Source: CAD feature listing. Evaluate the final solid. Frame: model axes, mm. Face numbers are marked on the shaded views. A direction names the side the tool comes from. Coordinates: 2 decimals unless noted, no trailing zeros. Loops run counter-clockwise (first coordinate to the right, second up) from the corner with the lowest first, then second, coordinate; pieces in that order, holes last. Notation, with made-up numbers: (71, 50) -> (104, 50) arc R13 cw to (104, 62) -> close; hole circle Ø6 at (-22, 62.5). An arc over 180 degrees is marked (long way). One line per question, with ' | ' between items. Start each with the question number.
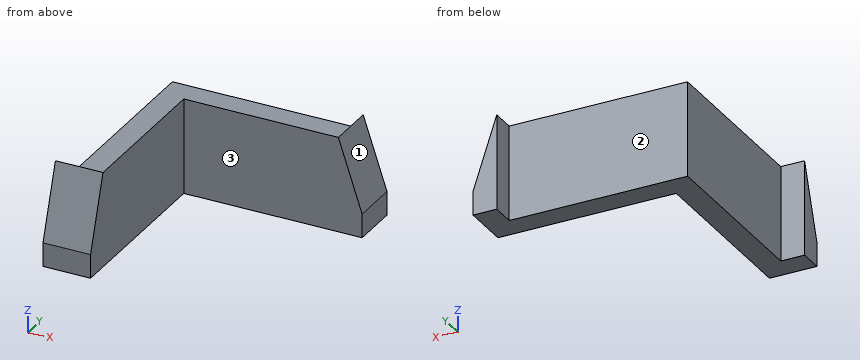
```python
from build123d import *

# Parameters (mm, degrees)
F1_DEPTH = 25.4
F2_SIZE2 = 19.05
F2_SIZE  = 6.35
F5_DEPTH = 6.35
F6_DEPTH = 6.35


with BuildPart() as f1:
    # F0 (on Top) → F1 (new body)
    with BuildSketch(Plane.XY):
        Polygon((-31.75, -22.225), (-25.4, -22.225), (-25.4, 25.4), (22.225, 25.4), (22.225, 31.75), (-31.75, 31.75), align=None)
    extrude(amount=F1_DEPTH)

    # F2
    f2_edges = [f1.edges().sort_by_distance(p)[0] for p in [
        (-28.575, -22.225, 25.4),
        (22.225, 28.575, 25.4),
    ]]
    f2_side = f1.faces().sort_by_distance((-28.575, -21.461678, 25.4))[0]
    chamfer(f2_edges, length=F2_SIZE, length2=F2_SIZE2, reference=f2_side)

    # F4 (on face) → F5 (join)
    with BuildSketch(Plane(origin=(0, 31.75, 0), x_dir=(-1, 0, 0), z_dir=(0, 1, 0))):
        Polygon((-15.875, 0), (-15.875, 25.4), (-22.225, 6.35), (-22.225, 0), align=None)
    extrude(amount=F5_DEPTH)

    # F3 (on face) → F6 (join)
    with BuildSketch(Plane(origin=(-31.75, 0, 0), x_dir=(0, -1, 0), z_dir=(-1, 0, 0))):
        Polygon((22.225, 6.35), (15.875, 25.4), (15.875, 0), (22.225, 0), align=None)
    extrude(amount=F6_DEPTH)


solid = f1.part
```
(1) Cut plane D-D, the plane z = 8.5. Return the cut outline in (x, y) (3 decimals).
(2) Cut plane C-C, the plane y = 14.5. Return the cut outline in (x, z), and give its area (3 significant figures).
(3) Cut plane A-A, the plane z = 4.5. Return the cut outline in (x, y) (3 decimals).
(4) Contact query for flat-ended pins moving along their axis: pin 1 Ø4 at (x, z) = (0, 11) entering from -Y; pin 2 Ø12.5 at (y, z) = (16.5, 8.5) entering from -X; pin 3 Ø3 at (y, z) = (24.5, 4) entering from +X (3 decimals); pin 4 Ø5 at (y, z) = (-11, 15.5) entering from +X. Output: stop coordinate, or through.
(5) Ray query, L1, parallel to X at y = -5, z = 22; L2, parallel to Y at x = 8, z = 19.5; L3, parallel to Y at x = -33.5, z = 5.75 (3 decimals). Return the intervals inside material, ascending.
(6) Cut plane B-B, the plane x = -29. Return the cut outline in (y, z) (3 decimals).
(7) Access query for the marked faces 1, 2 and 3. Directions: +Z, -Z, +X, -X, +Y, -Y. A direction counts if a zero-diameter tool reaches every point of the face in a straight line with its end or side. Return the directions, or none.
Here are the results:
1) outline: (-38.1, -21.508) -> (-25.4, -21.508) -> (-25.4, 25.4) -> (21.508, 25.4) -> (21.508, 38.1) -> (15.875, 38.1) -> (15.875, 31.75) -> (-31.75, 31.75) -> (-31.75, -15.875) -> (-38.1, -15.875) -> close
2) outline: (-31.75, 0) -> (-25.4, 0) -> (-25.4, 25.4) -> (-31.75, 25.4) -> close | area: 161 mm2
3) outline: (-38.1, -22.225) -> (-25.4, -22.225) -> (-25.4, 25.4) -> (22.225, 25.4) -> (22.225, 38.1) -> (15.875, 38.1) -> (15.875, 31.75) -> (-31.75, 31.75) -> (-31.75, -15.875) -> (-38.1, -15.875) -> close
4) pin 1: stops at y = 25.4 | pin 2: stops at x = -31.75 | pin 3: stops at x = 22.225 | pin 4: stops at x = -25.4
5) L1: x = -31.75 to -25.4 | L2: y = 25.4 to 31.75 | L3: y = -22.225 to -15.875
6) outline: (-22.225, 0) -> (31.75, 0) -> (31.75, 25.4) -> (-15.875, 25.4) -> (-22.225, 6.35) -> close
7) face 1: +Z, +X, +Y, -Y | face 2: +Z, -Z, -X, +Y | face 3: +Z, -Z, +X, -Y
